Source: CAD feature listing. Evaluate the final solid. Frame: model axes, mm. Round coordinates to 2 decimals unless told otherwise and drop trailing zeros. Order: outer loops, then holes, each group sorted by start corner. A loop starts at its lowest first (then second) coordinate and runs counter-clockwise, first axis right, second up. Notation, with made-up numbers: (-9.75, 83.25) -> (30.25, 83.25) arc R23 ccw to (30.25, 115.25) -> close; hole circle Ø5 at (-29.75, -34.75). An arc over 180 degrees is marked (long way). Answer as CSV lines item,"result".
from build123d import *

# Parameters (mm, degrees)
SKETCH1_W           = 46.6
SKETCH1_H           = 98.55
BOSS_EXTRUDE1_DEPTH = 1.65
SKETCH3_W           = 1.65
SKETCH3_H           = 95.25
BOSS_EXTRUDE2_DEPTH = 1.65
SKETCH2_W           = 1.65
SKETCH2_H           = 1.65
CUT_EXTRUDE1_DEPTH  = 1.65
SKETCH4_W           = 43.3
SKETCH4_H           = 1.65
CUT_EXTRUDE2_DEPTH  = 1.65


with BuildPart() as part:
    # Sketch1 → Boss-Extrude1 (new body)
    with BuildSketch(Plane.XY):
        Rectangle(SKETCH1_W, SKETCH1_H)
    extrude(amount=BOSS_EXTRUDE1_DEPTH)

    # Sketch3 → Boss-Extrude2 (add)
    with BuildSketch(Plane.ZY.offset(23.3)):
        with Locations((0.825, 0)):
            Rectangle(SKETCH3_W, SKETCH3_H)
    boss_extrude2 = extrude(amount=BOSS_EXTRUDE2_DEPTH)

    # Mirror1: Boss-Extrude2 across plane
    add(boss_extrude2.mirror(Plane(origin=(0, 0, 0), x_dir=(0, 0, 1), z_dir=(1, 0, 0))))

    # Sketch2 → Cut-Extrude1 (cut)
    with BuildSketch(Plane.XY.offset(1.65)):
        with Locations((20, -22.05)):
            Rectangle(SKETCH2_W, SKETCH2_H)
        with Locations((-20, -22.05)):
            Rectangle(SKETCH2_W, SKETCH2_H)
        with Locations((-22.05, -20)):
            Rectangle(SKETCH2_W, SKETCH2_H)
        with Locations((-22.05, 20)):
            Rectangle(SKETCH2_W, SKETCH2_H)
        with Locations((-20, 22.05)):
            Rectangle(SKETCH2_W, SKETCH2_H)
        with Locations((20, 22.05)):
            Rectangle(SKETCH2_W, SKETCH2_H)
        with Locations((22.05, 20)):
            Rectangle(SKETCH2_W, SKETCH2_H)
        with Locations((22.05, -20)):
            Rectangle(SKETCH2_W, SKETCH2_H)
    extrude(amount=-CUT_EXTRUDE1_DEPTH, mode=Mode.SUBTRACT)

    # Sketch4 → Cut-Extrude2 (cut)
    with BuildSketch(Plane.XZ.offset(49.275)):
        with Locations((0, 0.825)):
            Rectangle(SKETCH4_W, SKETCH4_H)
    cut_extrude2 = extrude(amount=-CUT_EXTRUDE2_DEPTH, mode=Mode.SUBTRACT)

    # Mirror2: Cut-Extrude2 across plane
    add(cut_extrude2.mirror(Plane.ZX), mode=Mode.SUBTRACT)


solid = part.part
1. Section query B-B on x = -14.5. Return loops of the section in (y, z) (3 decimals), and give its area (3 significant figures).
Results below:
outline,"(-47.625, 0) -> (47.625, 0) -> (47.625, 1.65) -> (-47.625, 1.65) -> close"
area,"157 mm2"
2. Line query: L1, parallel to Y at x = 22, z = 0.65 (3 decimals); L2, parallel to Y at x = -20.5, z = 0.45 (3 decimals); L3, parallel to Y at x = 1.5, z = 0.95 (3 decimals). Output: solid intervals per line, ascending. Write a range as [from, to].
Results below:
L1,"[-49.275, -20.825], [-19.175, 19.175], [20.825, 49.275]"
L2,"[-47.625, -22.875], [-21.225, 21.225], [22.875, 47.625]"
L3,"[-47.625, 47.625]"
3. Section query A-A on z = 0.95. Give the number of separate pieces and of enclosed holes in the cut face, and give its area (3 significant figures).
Results below:
separate pieces,"1"
enclosed holes,"8"
area,"4,740 mm2"
4. Pin query (flat end, axial travel): pin 1 (0.8 mm diameter, centred on y = -48.5, z = 1, fed in from -X); pin 2 (0.5 mm diameter, centred on x = 20, z = 0.5, fed in from +Y) (3 decimals); pin 3 (0.5 mm diameter, centred on x = -1, z = 0.5, fed in from -Y) (3 decimals). Return the tip coordinate at first contact, or that it passes through.
Results below:
pin 1,"x = -23.3"
pin 2,"y = 47.625"
pin 3,"y = -47.625"
